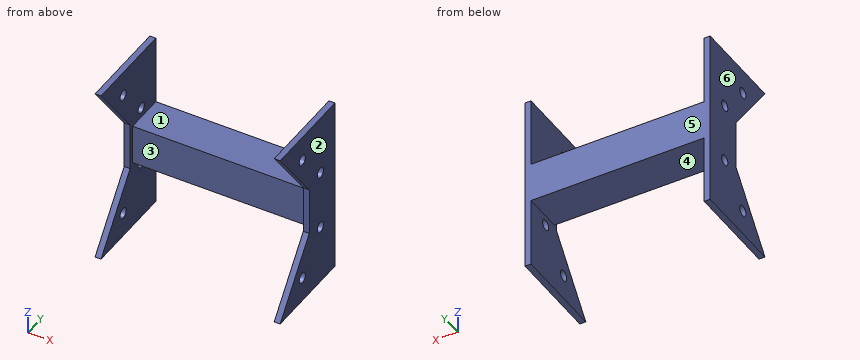
from build123d import *

# Parameters (mm, degrees)
BOSS_EXTRUDE1_DEPTH = 3.81
SKETCH3_W           = 25.4
SKETCH3_H           = 25.4
BOSS_EXTRUDE2_DEPTH = 55.245
SKETCH4_R           = 3.3782
CUT_EXTRUDE1_DEPTH  = 55.245
SCALE1_SCALE        = 1.02


with BuildPart() as part:
    # Sketch2 → Boss-Extrude1 (new body)
    with BuildSketch(Plane(origin=(0, 0, 0), x_dir=(0, 0, -1), z_dir=(1, 0, 0))):
        Polygon((15.24, 0), (-15.24, 0), (-57.15, -31.75), (-57.15, 27.94), (57.15, 27.94), (57.15, -31.75), align=None)
    boss_extrude1 = extrude(amount=BOSS_EXTRUDE1_DEPTH)

    # Sketch3 → Boss-Extrude2 (add)
    with BuildSketch(Plane(origin=(3.81, 0, 0), x_dir=(0, 0, -1), z_dir=(1, 0, 0))):
        with Locations((0, 15.24)):
            Rectangle(SKETCH3_W, SKETCH3_H)
    boss_extrude2 = extrude(amount=BOSS_EXTRUDE2_DEPTH)

    # Sketch4 → Cut-Extrude1 (cut)
    with BuildSketch(Plane.ZY):
        with Locations((19.05, 12.065)):
            Circle(SKETCH4_R)
        with Locations((41.275, -7.62)):
            Circle(SKETCH4_R)
        with Locations((-41.275, -7.62)):
            Circle(SKETCH4_R)
        with Locations((-19.05, 12.065)):
            Circle(SKETCH4_R)
    cut_extrude1 = extrude(amount=-CUT_EXTRUDE1_DEPTH, mode=Mode.SUBTRACT)

    # Mirror1: Boss-Extrude1, Boss-Extrude2, Cut-Extrude1 across plane
    add(boss_extrude1.mirror(Plane(origin=(59.055, 0, 0), x_dir=(0, 0, 1), z_dir=(1, 0, 0))))
    add(boss_extrude2.mirror(Plane(origin=(59.055, 0, 0), x_dir=(0, 0, 1), z_dir=(1, 0, 0))))
    add(cut_extrude1.mirror(Plane(origin=(59.055, 0, 0), x_dir=(0, 0, 1), z_dir=(1, 0, 0))), mode=Mode.SUBTRACT)


with BuildPart() as part_1:
    # Scale1: scaled about (59.055, 12.578988161, 0)
    add(part.part.scale(SCALE1_SCALE).moved(Location((-1.1811, -0.251579763, 0))))


solid = part_1.part
Source: CAD feature listing. Evaluate the final solid. Frame: model axes, mm. Face numbers are marked on the shaded views. A direction names the side the tool comes from. Coordinates: 2 decimals unless noted, no trailing zeros. Write each loop counter-clockwise with the first axis right and the second up, starting at its lowest first coordinate (ties: lowest second). Pieces come first, ordered by that corner, then holes. Notation, with made-up numbers: M 25,21 L 43,21 A20 ccw 43,35 Z; hole C 82,-24.5 d2. An arc over 180 degrees is marked long. Use a Markdown table: item, result.
1) Mould query, pull axis X, two halves, no side actions, for the marked faces 4, 5 and 6. Classes: pulls with the +X half, pulls with the -X half, needs draft (parallel to the pull), parting line crosses it, or undercut.
Conclusion:
| item | result |
|---|---|
| face 4 | undercut |
| face 5 | needs draft |
| face 6 | pulls with the -X half |
2) Section A-A, the plane z = 32. Output: boundary loops of the cut face in (x, y), then the cut area to 3 significant figures.
Conclusion:
| item | result |
|---|---|
| outline | M -1.18,-12.72 L 2.71,-12.72 L 2.71,28.25 L -1.18,28.25 Z; M 115.4,-12.72 L 119.29,-12.72 L 119.29,28.25 L 115.4,28.25 Z |
| area | 318 mm^2 |
3) Ray query, L1, parallel to X at y = 5.5, z = -22; L2, parallel to Y at x = 28, z = 2; L3, parallel to Z at x = 114, y = 22. Return the intervals inside material, ascending.
Conclusion:
| item | result |
|---|---|
| L1 | x = -1.18 to 2.71, 115.4 to 119.29 |
| L2 | y = 2.34 to 28.25 |
| L3 | z = -12.95 to 12.95 |
4) Section D-D, the plane y = -16. Output: boundary loops of the cut face in (x, z).
Conclusion:
| item | result |
|---|---|
| outline | M -1.18,-58.29 L 2.71,-58.29 L 2.71,-36.33 L -1.18,-36.33 Z; M -1.18,36.33 L 2.71,36.33 L 2.71,58.29 L -1.18,58.29 Z; M 115.4,-58.29 L 119.29,-58.29 L 119.29,-36.33 L 115.4,-36.33 Z; M 115.4,36.33 L 119.29,36.33 L 119.29,58.29 L 115.4,58.29 Z |
5) Section C-C, the plane z = 19. Output: boundary loops of the cut face in (x, y), then the cut area to 3 significant figures.
Conclusion:
| item | result |
|---|---|
| outline | M -1.18,-2.87 L 2.71,-2.87 L 2.71,8.64 L -1.18,8.64 Z; M -1.18,15.47 L 2.71,15.47 L 2.71,28.25 L -1.18,28.25 Z; M 115.4,-2.87 L 119.29,-2.87 L 119.29,8.64 L 115.4,8.64 Z; M 115.4,15.47 L 119.29,15.47 L 119.29,28.25 L 115.4,28.25 Z |
| area | 189 mm^2 |
6) First-contact query: pin 1 Ø20.5 at (x, z) = (80.5, 3.5) entering from -Y; pin 2 Ø6 at (x, y) = (39.5, 20.5) entering from -Z; pin 3 Ø4.5 at (x, z) = (0.5, -1) entering from -Y. Flat tips, straight axial feed; report the tip coordinate or a pass-through.
Conclusion:
| item | result |
|---|---|
| pin 1 | stops at y = 2.34 |
| pin 2 | stops at z = -12.95 |
| pin 3 | stops at y = -0.25 |
7) Reachability of the marked faces 1, 2 and 3 from +Z, -Z, +X, -X, +Y, -Y: full face, straight path, thin tool, end or side. Return the list, or none.
Conclusion:
| item | result |
|---|---|
| face 1 | +Z, +Y, -Y |
| face 2 | +Z, -Z, +X, +Y, -Y |
| face 3 | +Z, -Z, -Y |
8) Section B-B, the plane y = 14. Output: boundary loops of the cut face in (x, z), then the cut area to 3 significant figures.
Conclusion:
| item | result |
|---|---|
| outline | M -1.18,-58.29 L 2.71,-58.29 L 2.71,-22.28 L -1.18,-22.28 Z; M -1.18,-16.59 L 2.71,-16.59 L 2.71,-12.95 L 115.4,-12.95 L 115.4,-16.59 L 119.29,-16.59 L 119.29,16.59 L 115.4,16.59 L 115.4,12.95 L 2.71,12.95 L 2.71,16.59 L -1.18,16.59 Z; M -1.18,22.28 L 2.71,22.28 L 2.71,58.29 L -1.18,58.29 Z; M 115.4,-58.29 L 119.29,-58.29 L 119.29,-22.28 L 115.4,-22.28 Z; M 115.4,22.28 L 119.29,22.28 L 119.29,58.29 L 115.4,58.29 Z |
| area | 3,740 mm^2 |
